The model under review builds one solid part; all positions refer to its coordinate system, in mm. Face numbers are marked on the shaded views. A direction names the side the tool comes from. Give positions to 0.01 mm unless a question says otherwise; leave off trailing zeros. Order: outer loops, then holes, each group sorted by start corner. A loop starts at its lowest first (then second) coordinate and runs counter-clockwise, first axis right, second up. Notation, with made-up numbers: (-10.5, 77) - (23.5, 77) arc R11 ccw to (23.5, 96) - close; hole circle Ø7 at (28.5, 47.5). An arc over 180 degrees is marked (long way). Put each result on its own line as item: value.
```python
from build123d import *

# Parameters (mm, degrees)
F1_DEPTH = 20
F2_W     = 20
F2_H     = 20
F3_DEPTH = 5
F4_W     = 20
F4_H     = 20
F5_DEPTH = 5


with BuildPart() as f1:
    # F0 (on Right) → F1 (new body)
    with BuildSketch(Plane.YZ):
        Polygon((20, 15), (0, 5), (0, 0), (20, 0), align=None)
    extrude(amount=F1_DEPTH)

    # F2 (on Right) → F3 (join)
    with BuildSketch(Plane.YZ):
        with Locations((10, 10)):
            Rectangle(F2_W, F2_H)
    extrude(amount=F3_DEPTH)

    # F4 (on face) → F5 (join)
    with BuildSketch(Plane.YZ.offset(20)):
        with Locations((10, 10)):
            Rectangle(F4_W, F4_H)
    extrude(amount=F5_DEPTH)


solid = f1.part
```
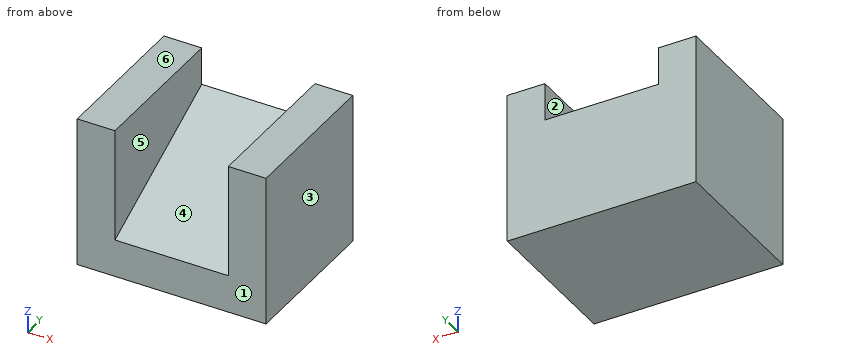
(1) Wall thickness on L1, parallel to X at y = 2.75, z = 10.5; L2, parallel to Z at x = 6.5, y = 13.5; L3, parallel to Z at x = 13.75, y = 14.75 (3 decimals): over which ranges is each line inside the solid? List them lowest first.
The answers:
L1: 0 to 5, 20 to 25
L2: 0 to 11.75
L3: 0 to 12.375
(2) Take a section at A-A, the plane z = 7.5. Write out the cut boundary in (x, y), then the cut area to 3 significant figures.
The answers:
outline: (0, 0) - (5, 0) - (5, 5) - (20, 5) - (20, 0) - (25, 0) - (25, 20) - (0, 20) - close
area: 425 mm^2
(3) For the marked faces 5 and 6, list the 3-axis set-ups (+Z, -Z, +X, -X, +Y, -Y) from which the entire face can be reached by the end or side of a thin tool; tool diameter is ignored.
The answers:
face 5: +Z, -Y
face 6: +Z, +X, -X, +Y, -Y
(4) Take a section at D-D, the plane x = 8.5. Write out the cut boundary in (y, z).
The answers:
outline: (0, 0) - (20, 0) - (20, 15) - (0, 5) - close
(5) Take a section at C-C, the plane z = 17.75. Write out the cut boundary in (x, y), then the cut area to 3 significant figures.
The answers:
outline: (0, 0) - (5, 0) - (5, 20) - (0, 20) - close; (20, 0) - (25, 0) - (25, 20) - (20, 20) - close
area: 200 mm^2
(6) Take a section at B-B, the plane y = 3.5. Write out the cut boundary in (x, z).
The answers:
outline: (0, 0) - (25, 0) - (25, 20) - (20, 20) - (20, 6.75) - (5, 6.75) - (5, 20) - (0, 20) - close
(7) The part is to be moulded in two halves that separate along X. For the marked faces 1, 2, 3 and 4, say which applies: pulls with the +X half, pulls with the -X half, needs draft (parallel to the pull), parting line crosses it, or undercut.
The answers:
face 1: needs draft
face 2: undercut
face 3: pulls with the +X half
face 4: undercut
(8) Clearance check with a flat-ended pin moving along its axis: pin 1 Ø1 at (x, z) = (12, 7.5) entering from -Y. State where the tip first meets the part, or that it passes through.
The answers:
pin 1: y = 4
